```python
from build123d import *

# Parameters (mm, degrees)
MAIN_STOCK_START             = 2.248090434
SKETCH_1_W                   = 49.95
SKETCH_1_H                   = 4
MAIN_STOCK_DEPTH             = 8.851909566
SKETCH_2_R                   = 0.8
FRAME_2XD1P6_THROUGH_DEPTH   = 51.615894766
SKETCH_3_R                   = 0.8
CORNER_L_2XD1P6_BLIND5_DEPTH = 5
CORNER_R_2XD1P6_BLIND5_START = -5
SKETCH_4_R                   = 0.8
CORNER_R_2XD1P6_BLIND5_DEPTH = 5


with BuildPart() as part:
    # 草图1 → Main_Stock (new body)
    with BuildSketch(Plane.XY.offset(MAIN_STOCK_START)):
        with Locations((24.675, -2.3)):
            Rectangle(SKETCH_1_W, SKETCH_1_H)
    extrude(amount=MAIN_STOCK_DEPTH)

    # 草图2 → Frame_2xD1p6_Through (cut, through all)
    with BuildSketch(Plane.XY.offset(11.1)):
        with Locations((12, -2.3)):
            Circle(SKETCH_2_R)
        with Locations((37.35, -2.3)):
            Circle(SKETCH_2_R)
    extrude(amount=-FRAME_2XD1P6_THROUGH_DEPTH, mode=Mode.SUBTRACT)

    # 草图3 → Corner_L_2xD1p6_Blind5 (cut)
    with BuildSketch(Plane.ZY.offset(0.3)):
        with Locations((5.1, -2.3)):
            Circle(SKETCH_3_R)
        with Locations((9.1, -2.3)):
            Circle(SKETCH_3_R)
    extrude(amount=-CORNER_L_2XD1P6_BLIND5_DEPTH, mode=Mode.SUBTRACT)

    # 草图4 → Corner_R_2xD1p6_Blind5 (cut)
    with BuildSketch(Plane(origin=(49.65, 0, 0), x_dir=(0, 0, -1), z_dir=(1, 0, 0)).offset(CORNER_R_2XD1P6_BLIND5_START)):
        with Locations(Location((-5.1, -2.3, 0), (0, 0, 180))):
            Circle(SKETCH_4_R)
        with Locations(Location((-9.1, -2.3, 0), (0, 0, 180))):
            Circle(SKETCH_4_R)
    extrude(amount=CORNER_R_2XD1P6_BLIND5_DEPTH, mode=Mode.SUBTRACT)


solid = part.part
```
Verification items for the finished model (mm, model axes). A direction names the side the tool comes from. Give positions to 0.01 mm unless a question says otherwise; leave off trailing zeros. Order: outer loops, then holes, each group sorted by start corner. A loop starts at its lowest first (then second) coordinate and runs counter-clockwise, first axis right, second up. Notation, with made-up numbers: (-8.5, 39) -> (38.5, 39) arc R19 cw to (38.5, 55) -> close; hole circle Ø4 at (38.25, 57). An arc over 180 degrees is marked (long way). Use a Markdown table: item, result.
1) Section check C-C, the plane z = 5.1. Record the boundary of the cut face in (x, y), then the cut area to 3 significant figures.
Results:
| item | result |
|---|---|
| outline | (-0.3, -4.3) -> (49.65, -4.3) -> (49.65, -3.1) -> (44.65, -3.1) -> (44.65, -1.5) -> (49.65, -1.5) -> (49.65, -0.3) -> (-0.3, -0.3) -> (-0.3, -1.5) -> (4.7, -1.5) -> (4.7, -3.1) -> (-0.3, -3.1) -> close; hole circle Ø1.6 at (12, -2.3); hole circle Ø1.6 at (37.35, -2.3) |
| area | 180 mm² |
2) Section check A-A, the plane x = 37.35. Record the boundary of the cut face in (y, z).
Results:
| item | result |
|---|---|
| outline | (-4.3, 2.25) -> (-3.1, 2.25) -> (-3.1, 11.1) -> (-4.3, 11.1) -> close; (-1.5, 2.25) -> (-0.3, 2.25) -> (-0.3, 11.1) -> (-1.5, 11.1) -> close |
3) Section check B-B, the plane y = -2.3. Record the boundary of the cut face in (x, z), then the cut area to 3 significant figures.
Results:
| item | result |
|---|---|
| outline | (-0.3, 2.25) -> (11.2, 2.25) -> (11.2, 11.1) -> (-0.3, 11.1) -> (-0.3, 9.9) -> (4.7, 9.9) -> (4.7, 8.3) -> (-0.3, 8.3) -> (-0.3, 5.9) -> (4.7, 5.9) -> (4.7, 4.3) -> (-0.3, 4.3) -> close; (12.8, 2.25) -> (36.55, 2.25) -> (36.55, 11.1) -> (12.8, 11.1) -> close; (38.15, 2.25) -> (49.65, 2.25) -> (49.65, 4.3) -> (44.65, 4.3) -> (44.65, 5.9) -> (49.65, 5.9) -> (49.65, 8.3) -> (44.65, 8.3) -> (44.65, 9.9) -> (49.65, 9.9) -> (49.65, 11.1) -> (38.15, 11.1) -> close |
| area | 382 mm² |
4) Material ranges on probe 1 along Z at (x, y) = (47.05, -2.3); probe 2 along Y at (x, z) = (47.7, 9.1); probe 3 along Z at (x, y) = (45, -2.7), recorded low to high.
Results:
| item | result |
|---|---|
| probe 1 | 2.25 to 4.3, 5.9 to 8.3, 9.9 to 11.1 |
| probe 2 | -4.3 to -3.1, -1.5 to -0.3 |
| probe 3 | 2.25 to 4.41, 5.79 to 8.41, 9.79 to 11.1 |
5) Tool access check on faces 4 (the flat face through (24, -2, 2.248)), 5 (the cylindrical face through (47.115, -2.54, 5.863)), 6 (the cylindrical face through (2.16, -1.76, 8.51)). Record the directions out of +Z, -Z, +X, -X, +Y, -Y that give a thin tool (end or side, any length) a straight path to the whole face; none if there is none.
Results:
| item | result |
|---|---|
| face 4 | -Z, +X, -X, +Y, -Y |
| face 5 | +X |
| face 6 | -X |
6) Mould release check, pull along Y, two halves, no side actions. Record for faces 1 (the flat face through (24, -4.3, 7)), 2 (the flat face through (24, -0.3, 7)), 3 (the flat face through (4.7, -2, 9)): pulls with the +Y half, pulls with the -Y half, needs draft (parallel to the pull), parting line crosses it, or undercut.
Results:
| item | result |
|---|---|
| face 1 | pulls with the -Y half |
| face 2 | pulls with the +Y half |
| face 3 | undercut |
7) Depth check by flat-ended pin: pin 1 Ø1.8 at (x, y) = (37.35, -2.3) entering from +Z; pin 2 Ø1 at (y, z) = (-2.3, 9.1) entering from -X; pin 3 Ø1.3 at (y, z) = (-2.3, 5.1) entering from +X. Enter the tip coordinate at first touch or a pass-through.
Results:
| item | result |
|---|---|
| pin 1 | z = 11.1 |
| pin 2 | x = 4.7 |
| pin 3 | x = 44.65 |
